Source: CAD feature listing. Evaluate the final solid. Frame: model axes, mm. Face numbers are marked on the shaded views. A direction names the side the tool comes from. Round coordinates to 2 decimals unless told otherwise and drop trailing zeros. Write each loop counter-clockwise with the first axis right and the second up, starting at its lowest first coordinate (ties: lowest second). Pieces come first, ordered by that corner, then holes. Notation, with made-up numbers: (-2.5, 46.25) - (17.5, 46.25) arc R6 cw to (17.5, 54.25) - close; hole circle Ø11 at (-31.5, 82.25). An arc over 180 degrees is marked (long way). Write item = value, one per line. Start each with the question number.
```python
from build123d import *

# Parameters (mm, degrees)
LINK1_BODY_DEPTH       = 8.5
TONGUE_CUT_DEPTH       = 37.789944278
TONGUE_CUT_DEPTH_BACK  = 37.789944278
SKETCH1_W              = 5.5
SKETCH1_H              = 15.998130079
SKETCH7_W              = 5.5
SKETCH7_H              = 7.8
BOSS_EXTRUDE1_DEPTH    = 8.5
SLOT_CUT_DEPTH         = 35.703602119
SLOT_CUT_DEPTH_BACK    = 35.703602119
SKETCH2_W              = 7.6
SKETCH2_H              = 18
PIN_HOLES_DEPTH        = 35.703602119
PIN_HOLES_DEPTH_BACK   = 35.703602119
SKETCH3_R              = 1.1
SKETCH3_R_2            = 1
SKETCH4_W              = 3.5
SKETCH4_H              = 2
GUIDE_BLOCK_1_DEPTH    = 2.5
CORD_GUIDES_DEPTH      = 36.473088391
CORD_GUIDES_DEPTH_BACK = 36.473088391
SKETCH6_R              = 0.6


with BuildPart() as part:
    # Link1_Outline → Link1_Body (new, symmetric)
    with BuildSketch(Plane.XY):
        with BuildLine():
            Line((-7.5, 0), (-7.5, 25))
            ThreePointArc((-7.5, 25), (0, 32.5), (7.5, 25))
            Line((7.5, 25), (7.5, 0))
            ThreePointArc((7.5, 0), (0, -7.5), (-7.5, 0))
        make_face()
    extrude(amount=LINK1_BODY_DEPTH, both=True)

    # Sketch1 → Tongue_Cut (cut, two sides: drawn at the far end of the back side and taken through both)
    with BuildSketch(Plane(origin=(7.5, 0, 0), x_dir=(0, 0, -1), z_dir=(1, 0, 0)).offset(-TONGUE_CUT_DEPTH_BACK)):
        with Locations((6.25, -0.00093496)):
            Rectangle(SKETCH1_W, SKETCH1_H)
        with Locations((-6.25, -0.00093496)):
            Rectangle(SKETCH1_W, SKETCH1_H)
    extrude(amount=TONGUE_CUT_DEPTH + TONGUE_CUT_DEPTH_BACK, mode=Mode.SUBTRACT)

    # Sketch7 → Boss-Extrude1 (add, symmetric)
    with BuildSketch(Plane.XY):
        with Locations((-4.75, 28.9)):
            Rectangle(SKETCH7_W, SKETCH7_H)
    extrude(amount=BOSS_EXTRUDE1_DEPTH, both=True)

    # Sketch2 → Slot_Cut (cut, two sides: drawn at the far end of the back side and taken through both)
    with BuildSketch(Plane(origin=(0, 0, 0), x_dir=(0, 0, -1), z_dir=(1, 0, 0)).offset(-SLOT_CUT_DEPTH_BACK)):
        with Locations((0, 26)):
            Rectangle(SKETCH2_W, SKETCH2_H)
    extrude(amount=SLOT_CUT_DEPTH + SLOT_CUT_DEPTH_BACK, mode=Mode.SUBTRACT)

    # Sketch3 → Pin_Holes (cut, two sides: drawn at the far end of the back side and taken through both)
    with BuildSketch(Plane.XY.offset(-PIN_HOLES_DEPTH_BACK)):
        Circle(SKETCH3_R)
        with Locations((0, 25)):
            Circle(SKETCH3_R_2)
    extrude(amount=PIN_HOLES_DEPTH + PIN_HOLES_DEPTH_BACK, mode=Mode.SUBTRACT)

    # Sketch4 → Guide_Block_1 (add, symmetric)
    with BuildSketch(Plane.XY):
        with Locations((8.75, 12.5)):
            Rectangle(SKETCH4_W, SKETCH4_H)
    extrude(amount=GUIDE_BLOCK_1_DEPTH, both=True)

    # Sketch6 → Cord_Guides (cut, two sides: drawn at the far end of the back side and taken through both)
    with BuildSketch(Plane(origin=(0, 0, 0), x_dir=(1, 0, 0), z_dir=(0, 1, 0)).offset(-CORD_GUIDES_DEPTH_BACK)):
        with Locations(Location((9, 0, 0), (0, 0, 90))):
            Circle(SKETCH6_R)
    extrude(amount=CORD_GUIDES_DEPTH + CORD_GUIDES_DEPTH_BACK, mode=Mode.SUBTRACT)


solid = part.part
```
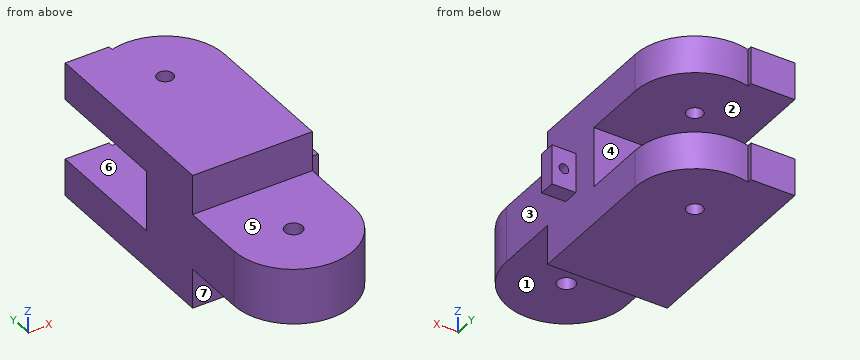
(1) Section A-A (z = 0). Return the cut outline in (x, y), plus the area to 3 significant figures.
(2) Reachability of the marked faces 5, 6 and 7 from +Z, -Z, +X, -X, +Y, -Y: full face, straight path, thin tool, end or side. Return the list, or none.
(3) Section B-B (x = 9). Return the cut outline in (y, z), plus the area to 3 significant figures.
(4) Pull-direction query (Z, two-part tool) for the marked faces 1, 2, 3 and 4; classes: +Z half, -Z half, draft (parallel to the pull), parting line (faces both ways), or undercut.
(5) Contact query for flat-ended pins moving along their axis: P1, Ø1.5, axis at x = 0, z = -6.5, coming from the -Y side; P2, Ø7.5, axis at x = -3, y = 0, coming from the -Z side; P3, Ø2.5, axis at x = -3.5, z = 1.5, coming from the +Y side; P4, Ø1.2, axis at x = 0, y = 25, coming from the +Z side. Output: stop coordinate, or through.
(6) Section C-C (y = 25.5). Return the cut outline in (x, z).
(7) Section D-D (z = -4.75). Return the cut outline in (x, y).
(8) Ray query, L1, parallel to X at y = 25, z = 6; L2, parallel to Y at x = 0, z = 5.6; L3, parallel to Z at x = -0.5, y = 29. Return the intervals inside material, ascending. Write a range as from..to.
Solution:
q1.outline = (-7.5, 0) arc R7.5 ccw to (7.5, 0) - (7.5, 11.5) - (8.4, 11.5) - (8.4, 13.5) - (7.5, 13.5) - (7.5, 17) - (-7.5, 17) - close; (9.6, 11.5) - (10.5, 11.5) - (10.5, 13.5) - (9.6, 13.5) - close; hole circle Ø2.2 at (0, 0)
q1.area = 343 mm^2
q2.face_5 = +Z, +X, -X, -Y
q2.face_6 = +X, -X, +Y
q2.face_7 = -Z, +X, -X, -Y
q3.outline = (11.5, -2.5) - (13.5, -2.5) - (13.5, -0.6) - (11.5, -0.6) - close; (11.5, 0.6) - (13.5, 0.6) - (13.5, 2.5) - (11.5, 2.5) - close
q3.area = 7.60 mm^2
q4.face_1 = -Z half
q4.face_2 = undercut
q4.face_3 = draft
q4.face_4 = undercut
q5.P1 = 8
q5.P2 = -3.5
q5.P3 = 17
q5.P4 = through
q6.outline = (-7.5, -8.5) - (-0.87, -8.5) - (-0.87, -3.8) - (-7.5, -3.8) - close; (-7.5, 3.8) - (-0.87, 3.8) - (-0.87, 8.5) - (-7.5, 8.5) - close; (0.87, -8.5) - (7.48, -8.5) - (7.48, -3.8) - (0.87, -3.8) - close; (0.87, 3.8) - (7.48, 3.8) - (7.48, 8.5) - (0.87, 8.5) - close
q7.outline = (-7.5, 8) - (7.5, 8) - (7.5, 25) arc R7.5 ccw to (-2, 32.23) - (-2, 32.8) - (-7.5, 32.8) - close; hole circle Ø2 at (0, 25)
q8.L1 = -7.5..-1, 1..7.5
q8.L2 = 8..24, 26..32.5
q8.L3 = -8.5..-3.8, 3.8..8.5
